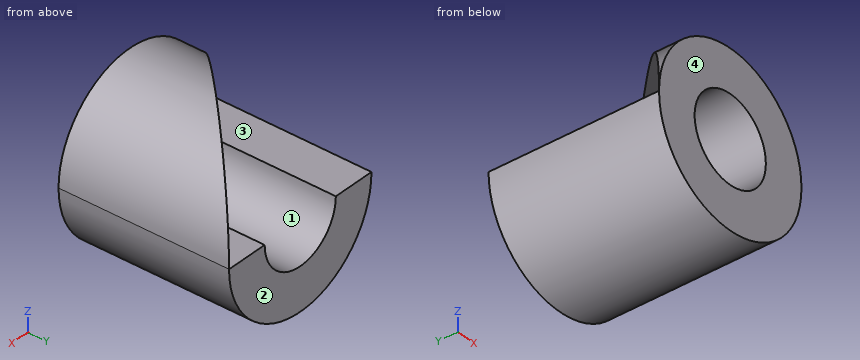
```python
from build123d import *

# Parameters (mm, degrees)
SKETCH1_W          = 10
SKETCH1_H          = 20
SKETCH2_R          = 5
CUT_EXTRUDE4_DEPTH = 20
CUT_EXTRUDE5_DEPTH = 10


with BuildPart() as part:
    # Sketch1 → Revolve1 (revolve)
    with BuildSketch(Plane.XY):
        with Locations((5, 10)):
            Rectangle(SKETCH1_W, SKETCH1_H)
    revolve(axis=Axis((0, 0, 0), (0, 1, 0)))

    # Sketch2 → Cut-Extrude4 (cut)
    with BuildSketch(Plane(origin=(0, 20, 0), x_dir=(1, 0, 0), z_dir=(0, 1, 0))):
        Circle(SKETCH2_R)
    extrude(amount=-CUT_EXTRUDE4_DEPTH, mode=Mode.SUBTRACT)

    # Sketch4 → Cut-Extrude5 (cut)
    with BuildSketch(Plane.XY):
        Polygon((10, 20), (-10, 0), (-10, 20), align=None)
    extrude(amount=CUT_EXTRUDE5_DEPTH, mode=Mode.SUBTRACT)


solid = part.part
```
Source: CAD feature listing. Evaluate the final solid. Frame: model axes, mm. Face numbers are marked on the shaded views. A direction names the side the tool comes from. Give positions to 0.01 mm unless a question says otherwise; leave off trailing zeros. Order: outer loops, then holes, each group sorted by start corner. A loop starts at its lowest first (then second) coordinate and runs counter-clockwise, first axis right, second up.
(1) Section query D-D (x = 5.5). Return the cut outline in (y, z), plus the area to 3 significant figures.
(2) Contact query for flat-ended pins moving along their axis: P1, Ø4, axis at y = 5.5, z = 5, coming from the -X side; P2, Ø2, axis at x = 2, y = 12.5, coming from the +Z side; P3, Ø4, axis at x = 8, y = 17, coming from the +Z side. Output: stop coordinate, or through.
(3) Section query A-A (x = 1.5). Return the cut outline in (y, z), plus the area to 3 significant figures.
(4) Section query C-C (y = 16.25). Return the cut outline in (x, z).
(5) Material intervals for line 1 along Z through (x, y) = (0, 6); line 2 along Z through (x, y) = (0, 15); line 3 along X through (y, z) = (7.25, -4), sorted ascending.
(6) Access query for the marked faces 3 and 4. Directions: +Z, -Z, +X, -X, +Y, -Y. A direction counts if a zero-diameter tool reaches every point of the face in a straight line with its end or side. Return the directions, or none.
(7) Pull-direction query (X, two-part tool) for the marked faces 1 and 2; classes: +X half, -X half, draft (parallel to the pull), parting line (faces both ways), or undercut.
(8) Section query B-B (z = -1.75). Return the cut outline in (x, y), plus the area to 3 significant figures.
Outcome:
1. outline: (0, -8.35) - (20, -8.35) - (20, 0) - (15.5, 0) - (15.5, 8.35) - (0, 8.35) - close
1. area: 296 mm2
2. P1: stops at x = -6.5
2. P2: stops at z = 9.87
2. P3: stops at z = 7.86
3. outline: (0, -9.89) - (20, -9.89) - (20, -4.77) - (0, -4.77) - close; (0, 4.77) - (11.5, 4.77) - (11.5, 9.89) - (0, 9.89) - close
3. area: 161 mm2
4. outline: (-10, 0) arc R10 ccw (long way) to (6.25, 7.81) - (6.25, 0) - (5, 0) arc R5 cw to (-5, 0) - close
5. line 1: z = -10 to -5, 5 to 10
5. line 2: z = -10 to -5
5. line 3: x = -9.17 to -3, 3 to 9.17
6. face 3: +Z, -X, +Y
6. face 4: +Z, -Z, +X, -X, -Y
7. face 1: undercut
7. face 2: draft
8. outline: (-9.85, 0) - (-4.68, 0) - (-4.68, 20) - (-9.85, 20) - close; (4.68, 0) - (9.85, 0) - (9.85, 20) - (4.68, 20) - close
8. area: 206 mm2
